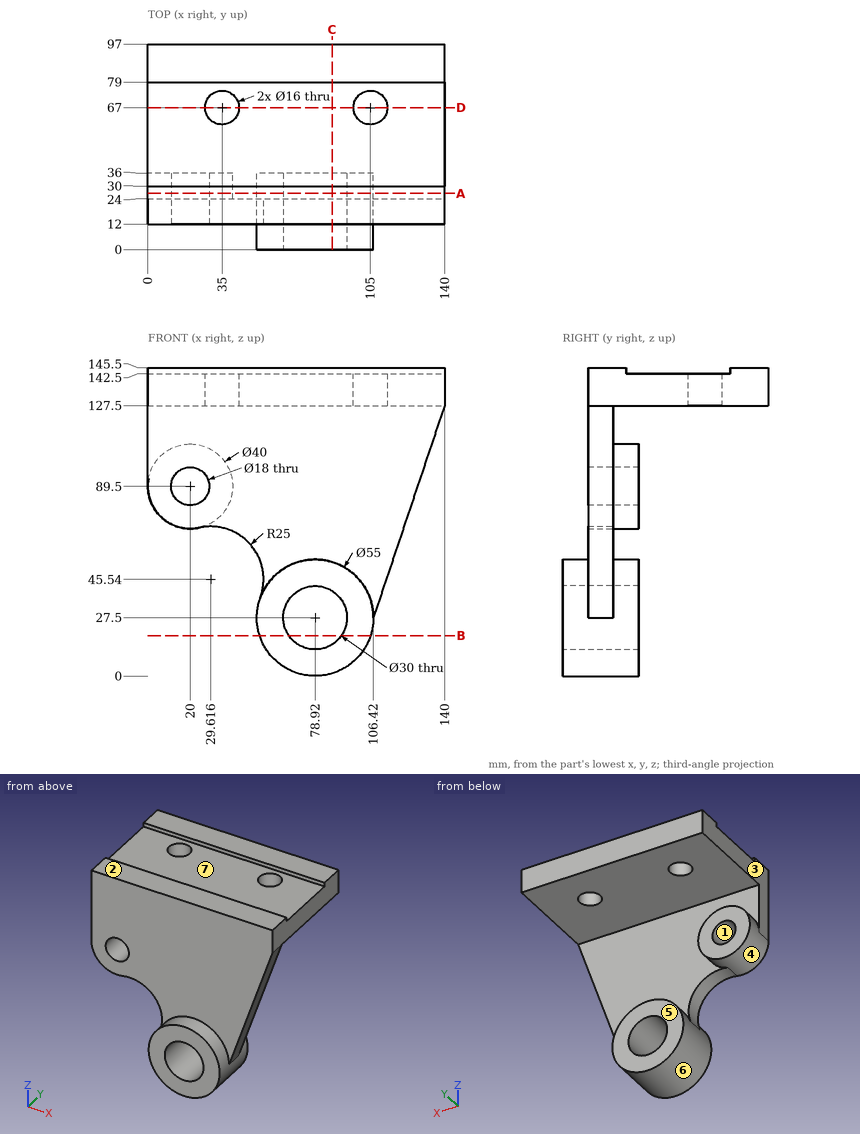
Design review of the part shown in the three views and the two pictorial views. Dimensions are in mm from the part's minimum x, y and z. A direction names the side the tool comes from. Give positions to 0.01 mm unless a question says otherwise; leave off trailing zeros. Write each loop counter-clockwise with the first axis right and the second up, starting at its lowest first coordinate (ties: lowest second). Pieces come first, ordered by that corner, then holes.
Item 1: Take a section at A-A (y = 26.5). Give the boundary of the cut face in (x, z).
Item 2: Wall thickness on probe 1 along X at (y, z) = (10, 27.5); probe 2 along Y at (x, z) = (35, 130.75); probe 3 along X at (y, z) = (27.5, 89.5): over which ranges is each line inside the solid? List them lowest first.
Item 3: The part is to be moulded in two halves that separate along X. For the marked faces 1, 2 and 3, say which applies: +X half, -X half, draft (parallel to the pull), parting line (faces both ways), or undercut.
Item 4: Take a section at C-C (x = 87). Give the boundary of the cut face in (y, z), and give its area (3 significant figures).
Item 5: Take a section at B-B (z = 19). Give the boundary of the cut face in (x, y), and give its area (3 significant figures).
Item 6: Take a section at D-D (y = 67). Give the boundary of the cut face in (x, z), and give its area (3 significant figures).
Item 7: Machinability: for the marked faces 4, 5, 6 and 7, which of the approach directions +Z, -Z, +X, -X, +Y, -Y give a long, thin tool a straight path to every point of the face, cutting with its end or side? Answer none if there is none.
Item 8: Insertion check: P1, Ø14.5, axis at x = 37.5, y = 57, coming from the +Z side; P2, Ø9.5, axis at x = 105, y = 67, coming from the -Z side; P3, Ø20.5, axis at x = 20, z = 89.5, coming from the -Y side; P4, Ø21, axis at x = 35, y = 67, coming from the -Z side. Each pin has a flat end and moves straight along its axis. Give the tip position at first contact, or say it passes through.
Established:
1. outline: circle Ø40 at (20, 89.5); (0, 127.5) - (140, 127.5) - (140, 145.5) - (0, 145.5) - close; circle Ø55 at (78.92, 27.5); hole circle Ø18 at (20, 89.5); hole circle Ø30 at (78.92, 27.5)
2. probe 1: x = 51.42 to 63.92, 93.92 to 106.42
2. probe 2: y = 12 to 59, 75 to 97
2. probe 3: x = 0 to 11, 29 to 40
3. face 1: undercut
3. face 2: draft
3. face 3: -X half
4. outline: (0, 1.21) - (36, 1.21) - (36, 14.86) - (0, 14.86) - close; (0, 40.14) - (36, 40.14) - (36, 53.79) - (24, 53.79) - (24, 127.5) - (97, 127.5) - (97, 145.5) - (79, 145.5) - (79, 142.5) - (30, 142.5) - (30, 145.5) - (12, 145.5) - (12, 53.79) - (0, 53.79) - close
4. area: 3,250 mm2
5. outline: (52.77, 0) - (66.56, 0) - (66.56, 36) - (52.77, 36) - close; (91.28, 0) - (105.07, 0) - (105.07, 36) - (91.28, 36) - close
5. area: 993 mm2
6. outline: (0, 127.5) - (27, 127.5) - (27, 142.5) - (0, 142.5) - close; (43, 127.5) - (97, 127.5) - (97, 142.5) - (43, 142.5) - close; (113, 127.5) - (140, 127.5) - (140, 142.5) - (113, 142.5) - close
6. area: 1,620 mm2
7. face 4: +Y
7. face 5: -Z, +X, -X, +Y
7. face 6: none
7. face 7: +Z, +X, -X
8. P1: stops at z = 142.5
8. P2: passes through
8. P3: stops at y = 12
8. P4: stops at z = 127.5
